```python
from build123d import *

# Parameters (mm, degrees)
BOSS_EXTRUDE1_DEPTH      = 0.915069
BOSS_EXTRUDE1_DEPTH_BACK = 2.834931
FILLET1_R                = 1.5
BOSS_EXTRUDE2_DEPTH      = 0.75


with BuildPart() as part:
    # Sketch1 → Boss-Extrude1 (new body, two sides)
    with BuildSketch(Plane.XY) as boss_extrude1_sk:
        with BuildLine():
            Line((7.72784891, 5.099738578), (7.72784891, 4.315453477))
            Line((7.72784891, 4.315453477), (6.47784891, 4.315453477))
            Line((6.47784891, 4.315453477), (6.47784891, 5.099738578))
            ThreePointArc((6.47784891, 5.099738578), (7.446291457, 10.050539659), (10.698263175, 13.90709152))
            Line((10.698263175, 13.90709152), (14.27784891, 15.955670445))
            ThreePointArc((14.27784891, 15.955670445), (17.77784891, 12.455670445), (21.27784891, 15.955670445))
            Line((21.27784891, 15.955670445), (24.857434644, 13.90709152))
            ThreePointArc((24.857434644, 13.90709152), (28.109406362, 10.050539659), (29.07784891, 5.099738578))
            Line((29.07784891, 5.099738578), (29.07784891, 4.315453477))
            Line((29.07784891, 4.315453477), (27.82784891, 4.315453477))
            Line((27.82784891, 4.315453477), (27.82784891, 5.099738578))
            ThreePointArc((27.82784891, 5.099738578), (26.841010044, 9.442734118), (24.074294629, 12.932826814))
            ThreePointArc((24.074294629, 12.932826814), (22.313278152, 13.328845303), (20.921800097, 12.179150343))
            ThreePointArc((20.921800097, 12.179150343), (17.77784891, 10.149738578), (14.633897723, 12.179150343))
            ThreePointArc((14.633897723, 12.179150343), (13.242419668, 13.328845303), (11.48140319, 12.932826814))
            ThreePointArc((11.48140319, 12.932826814), (8.714687776, 9.442734118), (7.72784891, 5.099738578))
        make_face()
    extrude(amount=BOSS_EXTRUDE1_DEPTH)
    extrude(boss_extrude1_sk.sketch, amount=-BOSS_EXTRUDE1_DEPTH_BACK)

    # Fillet1
    fillet1_edges = [part.edges().sort_by_distance(p)[0] for p in [
        (21.27784891, 15.955670445, -0.959931),
        (14.27784891, 15.955670445, -0.959931),
    ]]
    fillet(fillet1_edges, radius=FILLET1_R)

    # Sketch3 → Boss-Extrude2 (add)
    with BuildSketch(Plane.XY.offset(0.915069038)):
        with BuildLine():
            Line((12.579684297, 14.983819371), (10.698263175, 13.90709152))
            ThreePointArc((10.698263175, 13.90709152), (7.446291457, 10.050539659), (6.47784891, 5.099738578))
            Line((6.47784891, 5.099738578), (6.47784891, 4.315453477))
            Line((6.47784891, 4.315453477), (29.07784891, 4.315453477))
            Line((29.07784891, 4.315453477), (29.07784891, 5.099738578))
            ThreePointArc((29.07784891, 5.099738578), (28.909313649, 7.636891502), (28.109406362, 10.050539659))
            ThreePointArc((28.109406362, 10.050539659), (26.72021242, 12.178486343), (24.857434644, 13.90709152))
            Line((24.857434644, 13.90709152), (22.976013523, 14.983819371))
            ThreePointArc((22.976013523, 14.983819371), (21.80280977, 15.119540101), (20.895023154, 14.364059709))
            ThreePointArc((20.895023154, 14.364059709), (17.77784891, 12.455670445), (14.660674666, 14.364059709))
            ThreePointArc((14.660674666, 14.364059709), (13.75288805, 15.119540101), (12.579684297, 14.983819371))
        make_face()
    extrude(amount=BOSS_EXTRUDE2_DEPTH)


solid = part.part
```
Input: part model. Units: mm. Frame: model coordinates. A direction names the side the tool comes from. Coordinates: 2 decimals unless noted, no trailing zeros. Write each loop counter-clockwise with the first axis right and the second up, starting at its lowest first coordinate (ties: lowest second). Pieces come first, ordered by that corner, then holes. Notation, with made-up numbers: (-1.5, 70) -> (16.5, 70) arc R22 cw to (16.5, 102) -> close; hole circle Ø5 at (-36, -34). An arc over 180 degrees is marked (long way). Answer as a JSON object with one key per item and string values.
1. Access query for faces 1 (the face through (26.868, 9.386, -0.934)), 2 (the face through (18, 9, 1.665)). Directions: +Z, -Z, +X, -X, +Y, -Y. A direction counts if a zero-diameter tool reaches every point of the face in a straight line with its end or side. Return the directions, or none.
Result set:
{"face 1": "-Z, -Y", "face 2": "+Z, +X, -X, +Y, -Y"}
2. Section B-B on z = 0.05. Return the cut outline in (x, y).
Result set:
{"outline": "(6.48, 4.32) -> (7.73, 4.32) -> (7.73, 5.1) arc R10.05 cw to (11.48, 12.93) arc R2.05 cw to (14.63, 12.18) arc R3.45 ccw to (20.92, 12.18) arc R2.05 cw to (24.07, 12.93) arc R10.05 cw to (27.83, 5.1) -> (27.83, 4.32) -> (29.08, 4.32) -> (29.08, 5.1) arc R10.05 ccw to (24.86, 13.91) -> (22.98, 14.98) arc R1.5 ccw to (20.9, 14.36) arc R3.5 cw to (14.66, 14.36) arc R1.5 ccw to (12.58, 14.98) -> (10.7, 13.91) arc R10.05 ccw to (6.48, 5.1) -> close"}
3. Section C-C on x = 20.5. Return the cut outline in (y, z).
Result set:
{"outline": "(4.32, 0.92) -> (11.48, 0.92) -> (11.48, -2.83) -> (13.76, -2.83) -> (13.76, 1.67) -> (4.32, 1.67) -> close"}
4. Mould query, pull axis X, two halves, no side actions, for faces 3 (the face through (8.742, 9.499, -0.934)), 4 (the face through (18, 11, -2.835)), 5 (the face through (26.7, 12.2, 1.3)). Classes: released by +X, released by -X, zero draft, split by the parting line, or undercut.
Result set:
{"face 3": "undercut", "face 4": "zero draft", "face 5": "released by +X"}
5. Material intervals for line 1 (X direction, y = 12, z = -0.55); line 2 (Z direction, x = 22.5, y = 5); line 3 (X direction, y = 14, z = -0.05), sorted ascending. Write a range as from..to.
Result set:
{"line 1": "x = 8.67..10.47, 14.72..20.83, 25.08..26.88", "line 2": "z = 0.92..1.67", "line 3": "x = 10.86..14.88, 20.68..24.7"}
6. Section D-D on y = 6. Return the cut outline in (x, z).
Result set:
{"outline": "(6.46, -2.83) -> (7.77, -2.83) -> (7.77, 0.92) -> (27.79, 0.92) -> (27.79, -2.83) -> (29.09, -2.83) -> (29.09, 1.67) -> (6.46, 1.67) -> close"}
7. First-contact query: P1, Ø1, axis at y = 11, z = -1.5, coming from the -X side; P2, Ø2.5, axis at x = 21.5, y = 10.5, coming from the -Z side; P3, Ø0.9, axis at y = 5, z = -0.5, coming from the -X side. Flat tips, straight axial feed; report the tip coordinate or a pass-through.
Result set:
{"P1": "stops at x = 7.68", "P2": "stops at z = 0.92", "P3": "stops at x = 6.46"}
8. Section A-A on y = 7.5. Return the cut outline in (x, z).
Result set:
{"outline": "(6.62, -2.83) -> (8.02, -2.83) -> (8.02, 0.92) -> (27.54, 0.92) -> (27.54, -2.83) -> (28.94, -2.83) -> (28.94, 1.67) -> (6.62, 1.67) -> close"}
